```python
from build123d import *

# Parameters (mm, degrees)
F0_R     = 1.5875
F1_DEPTH = 0.79375


with BuildPart() as f1:
    # F0 (on Right) → F1 (new body)
    with BuildSketch(Plane.YZ):
        with BuildLine():
            ThreePointArc((-14.598681, -54.791494), (-2.692431, -57.966494), (9.213819, -54.791494))
            ThreePointArc((9.213819, -54.791494), (10.142302, -43.68735), (10.842757, -32.566494))
            ThreePointArc((10.842757, -32.566494), (6.835346, -18.163585), (11.595069, -3.991494))
            ThreePointArc((11.595069, -3.991494), (10.99943, 21.436396), (9.213819, 46.808506))
            ThreePointArc((9.213819, 46.808506), (-2.692431, 48.396006), (-14.598681, 46.808506))
            ThreePointArc((-14.598681, 46.808506), (-14.744138, 44.427464), (-14.882613, 42.046006))
            ThreePointArc((-14.882613, 42.046006), (-9.015448, 30.671057), (-15.83703, 19.841509))
            ThreePointArc((-15.83703, 19.841509), (-16.074209, -17.489202), (-14.598681, -54.791494))
        make_face()
        with Locations((-2.692431, -51.616494)):
            Circle(F0_R, mode=Mode.SUBTRACT)
        with Locations((-2.692431, 42.046006)):
            Circle(F0_R, mode=Mode.SUBTRACT)
        with Locations((6.832569, 10.296006)):
            Circle(F0_R, mode=Mode.SUBTRACT)
    extrude(amount=F1_DEPTH)


solid = f1.part
```
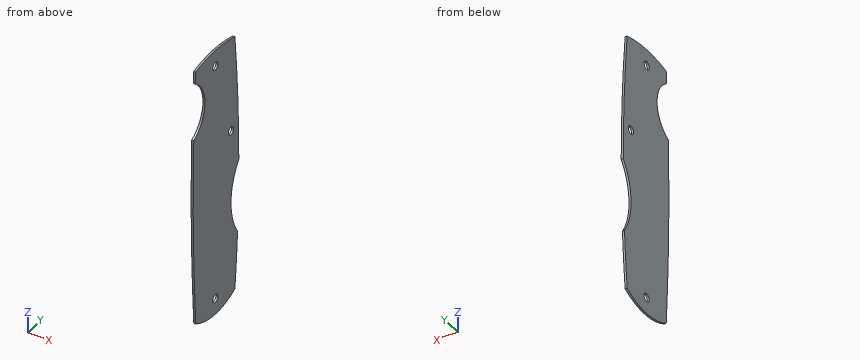
Build history of the part. All positions in model axes, mm. Round coordinates to 2 decimals unless told otherwise and drop trailing zeros. Loops run counter-clockwise (first coordinate to the right, second up) from the corner with the lowest first, then second, coordinate; pieces in that order, holes last.
Item 1: Saw through at D-D (z = -47). List the corners of the cut face in (x, y).
Item 2: Saw through at C-C (x = 0.45). List the corners of the cut face in (y, z) (1 decimal).
Item 3: Drill centre lines: line 1 along Z through (x, y) = (0.6, -2); line 2 along Z through (x, y) = (0.15, 5.5); line 3 along Y through (x, z) = (0.1, -0.5). Where is each one in solid material? Low to high.
Item 4: Saw through at A-A (y = -3). List the corners of the cut face in (x, z), then the cut area to 3 significant figures.
Item 5: Saw through at B-B (y = -11.25). List the corners of the cut face in (x, z), then the cut area to 3 significant figures.
Worked answers:
1. outline: (0, -15.05) - (0.79, -15.05) - (0.79, 9.89) - (0, 9.89) - close
2. outline: (-15.8, 19.8) arc R813.6 ccw to (-14.6, -54.8) arc R23.9 ccw to (9.2, -54.8) arc R543.1 ccw to (10.8, -32.6) arc R25.5 cw to (11.6, -4) arc R543.1 ccw to (9.2, 46.8) arc R45.4 ccw to (-14.6, 46.8) arc R813.6 ccw to (-14.9, 42) arc R12.9 cw to start; hole circle Ø3.2 at (-2.7, -51.6); hole circle Ø3.2 at (-2.7, 42); hole circle Ø3.2 at (6.8, 10.3)
3. line 1: z = -57.96 to -53.05, -50.19 to 40.62, 43.47 to 48.39
3. line 2: z = -56.52 to 9.43, 11.16 to 47.65
3. line 3: y = -16.18 to 11.58
4. outline: (0, -57.96) - (0.79, -57.96) - (0.79, -53.17) - (0, -53.17) - close; (0, -50.06) - (0.79, -50.06) - (0.79, 40.49) - (0, 40.49) - close; (0, 43.6) - (0.79, 43.6) - (0.79, 48.39) - (0, 48.39) - close
4. area: 79.5 mm2
5. outline: (0, -56.38) - (0.79, -56.38) - (0.79, 23.95) - (0, 23.95) - close; (0, 38.5) - (0.79, 38.5) - (0.79, 47.58) - (0, 47.58) - close
5. area: 71.0 mm2
